Build history of the part. All positions in model axes, mm. A direction names the side the tool comes from. Round coordinates to 2 decimals unless told otherwise and drop trailing zeros. Order: outer loops, then holes, each group sorted by start corner. A loop starts at its lowest first (then second) coordinate and runs counter-clockwise, first axis right, second up. Notation, with made-up numbers: (-17, 20) -> (-3, 20) arc R28 ccw to (-3, 48) -> close; hole circle Ø2 at (57, 74). An arc over 180 degrees is marked (long way). Write item = value, one per line.
from build123d import *
from build123d.topology import SkipClean

# Parameters (mm, degrees)
SKETCH1_R           = 1.6
SKETCH1_R_2         = 10.75
SKETCH1_R_3         = 7.75
BOSS_EXTRUDE1_DEPTH = 2
SKETCH1_3_R         = 10.75
SKETCH1_3_R_2       = 7.75
BOSS_EXTRUDE2_DEPTH = 5.5
FILLET1_R           = 5
CHAMFER1_SIZE       = 1


with BuildPart() as part:
    # Sketch1 → Boss-Extrude1 (new body)
    with BuildSketch(Plane.XY):
        with BuildLine():
            ThreePointArc((-1.946953154, -10.572221782), (-5.375, -9.309773091), (-8.182336061, -6.972221782))
            Line((-8.182336061, -6.972221782), (-10.617691454, -11.190381057))
            ThreePointArc((-10.617691454, -11.190381057), (-9.3, -16.10807251), (-4.382308546, -14.790381057))
            Line((-4.382308546, -14.790381057), (-1.946953154, -10.572221782))
        make_face()
        with Locations((-7.5, -12.990381057)):
            Circle(SKETCH1_R, mode=Mode.SUBTRACT)
        with BuildLine():
            Line((13.630127019, 13.60807251), (4.969872981, 18.60807251))
            ThreePointArc((4.969872981, 18.60807251), (2.238124419, 18.967714031), (0.052181527, 17.290381057))
            Line((0.052181527, 17.290381057), (-4.222818473, 9.885863854))
            ThreePointArc((-4.222818473, 9.885863854), (5.375, 9.309773091), (10.672818473, 1.285863854))
            Line((10.672818473, 1.285863854), (14.947818473, 8.690381057))
            ThreePointArc((14.947818473, 8.690381057), (15.307459994, 11.422129619), (13.630127019, 13.60807251))
        make_face()
        with Locations((3.169872981, 15.490381057)):
            Circle(SKETCH1_R, mode=Mode.SUBTRACT)
        with Locations((11.830127019, 10.490381057)):
            Circle(SKETCH1_R, mode=Mode.SUBTRACT)
        Circle(SKETCH1_R_2)
        Circle(SKETCH1_R_3, mode=Mode.SUBTRACT)
    extrude(amount=BOSS_EXTRUDE1_DEPTH)

    # Sketch1<3> → Boss-Extrude2 (add)
    with SkipClean():  # the faces are left unmerged after this step: merging them gives an invalid solid
        with BuildSketch(Plane.XY):
            with Locations(Location((0, 0, 0), (0, 0, 180))):
                Circle(SKETCH1_3_R)
            with Locations(Location((0, 0, 0), (0, 0, 180))):
                Circle(SKETCH1_3_R_2, mode=Mode.SUBTRACT)
        extrude(amount=-BOSS_EXTRUDE2_DEPTH)

    # Fillet1
    fillet1_edges = [part.edges().sort_by_distance(p)[0] for p in [
        (-8.182336061, -6.972221782, 1),
        (-4.222818473, 9.885863854, 1),
        (10.672818473, 1.285863854, 1),
        (-1.946953154, -10.572221782, 1),
    ]]
    fillet(fillet1_edges, radius=FILLET1_R)

    # Chamfer1
    chamfer1_edges = [part.edges().sort_by_distance(p)[0] for p in [
        (-10.166389113, -10.408702474, 2),
        (-9.3, -16.10807251, 2),
        (-3.931006206, -14.008702474, 2),
        (13.183745523, 5.63491708, 2),
        (15.307459994, 11.422129619, 2),
        (9.3, 16.10807251, 2),
        (2.238124419, 18.967714031, 2),
        (-1.711891422, 14.23491708, 2),
        (7.822542831, -7.373623509, 2),
        (-10.297016692, 3.08770906, 2),
        (-7.75, 0, 2),
        (-4.27948651, 10.135012665, 2),
        (-9.047037625, -7.26206095, 2),
        (-1.765610454, -11.465994887, 2),
        (10.916921691, 1.3613623, 2),
    ]]
    chamfer(chamfer1_edges, length=CHAMFER1_SIZE)


solid = part.part
Q1. Which spindle directions (+Z, -Z, +X, -X, +Y, -Y) get a long thin tool onto all of the face, cutting with end or side? Do faces 4 (the face through (-10.18, -3.46, -2.2)), 5 (the face through (2, 9, 2)). Say none if no direction does.
Check values:
face_4 = -Z
face_5 = +Z, +X, -X, +Y, -Y
Q2. Flat gauge pins, fed straight in: pin 1 (1.5 mm diameter, centred on x = -5, y = -5, fed in from +Z); pin 2 (6 mm diameter, centred on x = 11.5, y = 9, fed in from -Z); pin 3 (1.5 mm diameter, centred on x = -8, z = -1, fed in from -Y). Where does each tip first touch, or does it go through?
Check values:
pin_1 = 1.07
pin_2 = 0
pin_3 = -7.94
Q3. Cut at A-A, the plane z = -1.5. List the corners of the cut face in (x, y), and give its area (3 significant figures).
Check values:
outline = circle Ø21.5 at (0, 0); hole circle Ø15.5 at (0, 0)
area = 174 mm²
Q4. Cut at B-B, the plane z = 0.5. List the corners of the cut face in (x, y), and give its area (3 significant figures).
Check values:
outline = (-10.62, -11.19) arc R3.6 ccw to (-4.38, -14.79) -> (-3.48, -13.23) arc R5 cw to (0.58, -10.73) arc R10.75 ccw to (10.75, 0.05) arc R5 cw to (11.42, 2.58) -> (14.95, 8.69) arc R3.6 ccw to (13.63, 13.61) -> (4.97, 18.61) arc R3.6 ccw to (0.05, 17.29) -> (-3.48, 11.18) arc R5 cw to (-5.33, 9.34) arc R10.75 ccw to (-9.59, -4.86) arc R5 cw to (-9.72, -9.63) -> close; hole circle Ø3.2 at (-7.5, -12.99); hole circle Ø15.5 at (0, 0); hole circle Ø3.2 at (3.17, 15.49); hole circle Ø3.2 at (11.83, 10.49)
area = 358 mm²
Q5. Mould opens along X. For faces 1 (the face through (12.57, 9.07, 0.99)), 2 (the face through (-9.368, -16.068, 0.493)), 3 (the face through (14.719, 11.23, 1.618)) say: released by +X, released by -X, zero draft, split by the parting line, or undercut.
Check values:
face_1 = undercut
face_2 = split by the parting line
face_3 = released by +X
Q6. Probe probe 1 along Z at (x, y) = (6.5, 11); probe 2 along Y at (x, z) = (-5.25, 1.25); probe 3 along Y at (x, z) = (-6, -1). List the from-to ranges inside material, lowest first.
Check values:
probe_1 = 0 to 2
probe_2 = -15.47 to -6.04, 6.04 to 9.09
probe_3 = -8.92 to -4.91, 4.91 to 8.92
